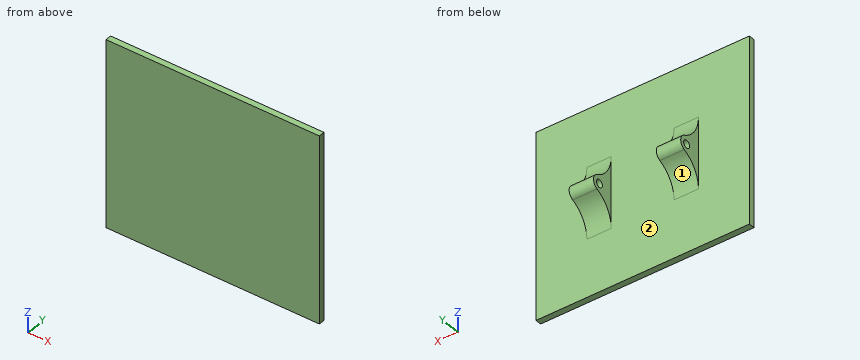
```python
from build123d import *
from build123d.topology import SkipClean

# Parameters (mm, degrees)
SKETCH1_W           = 20
SKETCH1_H           = 60
BOSS_EXTRUDE1_DEPTH = 5
SKETCH2_R           = 2.5
SKETCH2_R_2         = 1.25
BOSS_EXTRUDE2_DEPTH = 20
CUT_EXTRUDE1_START  = -29
SKETCH3_R           = 1.25
CUT_EXTRUDE1_DEPTH  = 29
SKETCH4_R           = 2.5
SKETCH4_R_2         = 1.25
BOSS_EXTRUDE3_DEPTH = 20
CUT_EXTRUDE2_START  = -29
SKETCH5_R           = 1.25
CUT_EXTRUDE2_DEPTH  = 29
BOSS_EXTRUDE4_START = 70
SKETCH7_R           = 1.25
BOSS_EXTRUDE4_DEPTH = 70
SKETCH8_W           = 20.6
SKETCH8_H           = 18.256228475
SKETCH8_W_2         = 16.7
SKETCH8_H_2         = 28.46865204
SKETCH8_H_3         = 26.746757763
CUT_EXTRUDE4_DEPTH  = 84
SKETCH9_W           = 45.88716948
SKETCH9_H           = 69.445914147
CUT_EXTRUDE5_DEPTH  = 115
FILLET1_R           = 10


with BuildPart() as part:
    # Sketch1 → Boss-Extrude1 (new body)
    with BuildSketch(Plane.XY):
        with Locations((10, 30)):
            Rectangle(SKETCH1_W, SKETCH1_H)
    extrude(amount=BOSS_EXTRUDE1_DEPTH)

    # Sketch2 → Boss-Extrude2 (add)
    with BuildSketch(Plane(origin=(20, 0, 0), x_dir=(0, 0, -1), z_dir=(1, 0, 0))):
        with Locations((-2.5, 60)):
            Circle(SKETCH2_R)
        with Locations((-2.5, 60)):
            Circle(SKETCH2_R_2, mode=Mode.SUBTRACT)
    extrude(amount=-BOSS_EXTRUDE2_DEPTH)

    # Sketch3 → Cut-Extrude1 (cut)
    with SkipClean():  # the faces are left unmerged after this step: merging them gives an invalid solid
        with BuildSketch(Plane.ZY.offset(CUT_EXTRUDE1_START)):
            with Locations(Location((2.5, 60, 0), (0, 0, 180))):
                Circle(SKETCH3_R)
        extrude(amount=CUT_EXTRUDE1_DEPTH, mode=Mode.SUBTRACT)

    # Sketch4 → Boss-Extrude3 (add)
    with BuildSketch(Plane.ZY):
        with Locations((2.5, 0)):
            Circle(SKETCH4_R)
        with Locations((2.5, 0)):
            Circle(SKETCH4_R_2, mode=Mode.SUBTRACT)
    extrude(amount=-BOSS_EXTRUDE3_DEPTH)

    # Sketch5 → Cut-Extrude2 (cut)
    with SkipClean():  # the faces are left unmerged after this step: merging them gives an invalid solid
        with BuildSketch(Plane(origin=(20, 0, 0), x_dir=(0, 0, -1), z_dir=(1, 0, 0)).offset(CUT_EXTRUDE2_START)):
            with Locations(Location((-2.5, 0, 0), (0, 0, 180))):
                Circle(SKETCH5_R)
        extrude(amount=CUT_EXTRUDE2_DEPTH, mode=Mode.SUBTRACT)

    # Sketch7 → Boss-Extrude4 (add)
    # profile 1 of 2: a face of its own
    with SkipClean():  # the faces are left unmerged after this step: merging them gives an invalid solid
        with BuildSketch(Plane.ZY.offset(BOSS_EXTRUDE4_START)):
            with BuildLine():
                Line((0, -5), (-27.5, -5))
                Line((-27.5, -5), (-27.5, -7))
                Line((-27.5, -7), (32.5, -7))
                Line((32.5, -7), (32.5, -5))
                Line((32.5, -5), (5, -5))
                Line((5, -5), (5, 0))
                ThreePointArc((5, 0), (2.5, -2.5), (0, 0))
                Line((0, 0), (0, -5))
            make_face()
        # profile 2 of 2: a face of its own
        with BuildSketch(Plane.ZY.offset(BOSS_EXTRUDE4_START)):
            with BuildLine():
                ThreePointArc((5, 0), (2.5, 2.5), (0, 0))
                ThreePointArc((0, 0), (2.5, -2.5), (5, 0))
            make_face()
            with Locations((2.5, 0)):
                Circle(SKETCH7_R, mode=Mode.SUBTRACT)
        extrude(amount=-BOSS_EXTRUDE4_DEPTH)

    # Sketch8 → Cut-Extrude4 (cut)
    with SkipClean():  # the faces are left unmerged after this step: merging them gives an invalid solid
        with BuildSketch(Plane(origin=(0, -5, 0), x_dir=(1, 0, 0), z_dir=(0, 1, 0))):
            with Locations((-35, -1.601019052)):
                Rectangle(SKETCH8_W, SKETCH8_H)
            with Locations((-8.35, -2.689028032)):
                Rectangle(SKETCH8_W_2, SKETCH8_H_2)
            with Locations((-61.65, -3.54997517)):
                Rectangle(SKETCH8_W_2, SKETCH8_H_3)
        extrude(amount=CUT_EXTRUDE4_DEPTH, mode=Mode.SUBTRACT)


with BuildPart() as cut_extrude4_piece_1:
    # of the separate pieces the step leaves, piece 1, a body of its own (cut_extrude4_pieces)
    add(part.part.solids().sort_by_distance((0, -5, 0))[0])

    # Fillet1
    # the kernel refuses this fillet: 10 mm, written as the material it adds along each edge
    with BuildSketch(Plane(origin=(-47.091098093, -5, 5), x_dir=(0, 0, 1), z_dir=(1, 0, 0))) as fillet1_piece_1_section:
        with BuildLine():
            CenterArc((8.956439237, -10), FILLET1_R, 90, 66.421821522)
            Line((-0.208712153, -6), (-1.125227292, -5.6))
            ThreePointArc((-1.125227292, -5.6), (-1, -5), (-1, 0))
            Line((-1, 0), (0, 1))
            Line((0, 1), (8.956439237, 1))
            Line((8.956439237, 1), (8.956439237, 0))
        make_face()
    fillet1_piece_1 = extrude(amount=30.391098093, mode=Mode.PRIVATE)
    fillet1_piece_1 = split(fillet1_piece_1, bisect_by=Plane(origin=(-45.3, -3.872690531, 7.347841943), z_dir=(-1, 0, 0)), keep=Keep.TOP, mode=Mode.PRIVATE)
    add(fillet1_piece_1)
    with BuildSketch(Plane(origin=(-24.7, -5, 5), x_dir=(0, 0, 1), z_dir=(1, 0, 0)), Plane(origin=(-53.3, -5, 5), x_dir=(0, 0, 1), z_dir=(1, 0, 0))) as fillet1_piece_2:
        with BuildLine():
            CenterArc((8.956439237, -10), FILLET1_R, 90, 66.421821522)
            Line((-0.208712153, -6), (-1.125227292, -5.6))
            ThreePointArc((-1.125227292, -5.6), (-1, -5), (-1, 0))
            Line((-1, 0), (0, 1))
            Line((0, 1), (8.956439237, 1))
            Line((8.956439237, 1), (8.956439237, 0))
        make_face()
    extrude(amount=8)
    with BuildSketch(Plane(origin=(-53.3, -5, 5), x_dir=(0, 0, 1), z_dir=(1, 0, 0))) as fillet1_piece_3_section:
        with BuildLine():
            CenterArc((8.956439237, -10), FILLET1_R, 90, 66.421821522)
            Line((-0.208712153, -6), (-1.125227292, -5.6))
            ThreePointArc((-1.125227292, -5.6), (-1, -5), (-1, 0))
            Line((-1, 0), (0, 1))
            Line((0, 1), (8.956439237, 1))
            Line((8.956439237, 1), (8.956439237, 0))
        make_face()
    fillet1_piece_3 = extrude(amount=30.391098093, mode=Mode.PRIVATE)
    fillet1_piece_3 = split(fillet1_piece_3, bisect_by=Plane(origin=(-24.7, -3.872690531, 7.347841943), z_dir=(1, 0, 0)), keep=Keep.TOP, mode=Mode.PRIVATE)
    add(fillet1_piece_3)
    with BuildSketch(Plane(origin=(-53.3, -5, 0), x_dir=(0, 0, -1), z_dir=(1, 0, 0)), Plane(origin=(-24.7, -5, 0), x_dir=(0, 0, -1), z_dir=(1, 0, 0))) as fillet1_piece_4:
        with BuildLine():
            CenterArc((8.956439237, 10), FILLET1_R, 203.578178478, 66.421821522)
            Line((-0.208712153, 6), (-1.125227292, 5.6))
            ThreePointArc((-1.125227292, 5.6), (-1, 5), (-1, 0))
            Line((-1, 0), (0, -1))
            Line((0, -1), (8.956439237, -1))
            Line((8.956439237, -1), (8.956439237, 0))
        make_face()
    extrude(amount=8)
    with BuildSketch(Plane(origin=(-53.3, -5, 0), x_dir=(0, 0, -1), z_dir=(1, 0, 0))) as fillet1_piece_5_section:
        with BuildLine():
            CenterArc((8.956439237, 10), FILLET1_R, 203.578178478, 66.421821522)
            Line((-0.208712153, 6), (-1.125227292, 5.6))
            ThreePointArc((-1.125227292, 5.6), (-1, 5), (-1, 0))
            Line((-1, 0), (0, -1))
            Line((0, -1), (8.956439237, -1))
            Line((8.956439237, -1), (8.956439237, 0))
        make_face()
    fillet1_piece_5 = extrude(amount=30.391098093, mode=Mode.PRIVATE)
    fillet1_piece_5 = split(fillet1_piece_5, bisect_by=Plane(origin=(-24.7, -3.872690531, -2.347841943), z_dir=(1, 0, 0)), keep=Keep.TOP, mode=Mode.PRIVATE)
    add(fillet1_piece_5)
    with BuildSketch(Plane(origin=(-47.091098093, -5, 0), x_dir=(0, 0, -1), z_dir=(1, 0, 0))) as fillet1_piece_6_section:
        with BuildLine():
            CenterArc((8.956439237, 10), FILLET1_R, 203.578178478, 66.421821522)
            Line((-0.208712153, 6), (-1.125227292, 5.6))
            ThreePointArc((-1.125227292, 5.6), (-1, 5), (-1, 0))
            Line((-1, 0), (0, -1))
            Line((0, -1), (8.956439237, -1))
            Line((8.956439237, -1), (8.956439237, 0))
        make_face()
    fillet1_piece_6 = extrude(amount=30.391098093, mode=Mode.PRIVATE)
    fillet1_piece_6 = split(fillet1_piece_6, bisect_by=Plane(origin=(-45.3, -3.872690531, -2.347841943), z_dir=(-1, 0, 0)), keep=Keep.TOP, mode=Mode.PRIVATE)
    add(fillet1_piece_6)


with BuildPart() as cut_extrude4_piece_2:
    # of the separate pieces the step leaves, piece 2, a body of its own (cut_extrude4_pieces)
    add(part.part.solids().sort_by_distance((20, 0, 0))[0])

    # Sketch9 → Cut-Extrude5 (cut)
    with BuildSketch(Plane(origin=(-16.7, 0, 0), x_dir=(0, 0, -1), z_dir=(1, 0, 0))):
        with Locations((-3.398393378, 29.722957074)):
            Rectangle(SKETCH9_W, SKETCH9_H)
    extrude(amount=CUT_EXTRUDE5_DEPTH, mode=Mode.SUBTRACT)


solid = cut_extrude4_piece_1.part
```
Verification items for the finished model (mm, model axes). Face numbers are marked on the shaded views. Give positions to 0.01 mm unless a question says otherwise; leave off trailing zeros. Order: outer loops, then holes, each group sorted by start corner. A loop starts at its lowest first (then second) coordinate and runs counter-clockwise, first axis right, second up. Notation, with made-up numbers: M -24.75,7.25 L 5.25,7.25 A19 ccw 5.25,12.25 Z; hole C -30,48.5 d10. An arc over 180 degrees is marked long. Return JSON: item names as keys, results as strings. Group by question number.
1) Section check D-D on z = 9.5. Record the cut outline in (x, y).
2) Section check A-A on z = 2.5. Record the cut outline in (x, y).
3) Go/stop test with flat-tipped pins: pin 1 Ø2 at (y, z) = (-3, 5) entering from -X; pin 2 Ø4 at (x, y) = (-49, 0) entering from +Z (3 decimals); pin 3 Ø3 at (y, z) = (0, 2.5) entering from +X; pin 4 Ø1.5 at (y, z) = (0, 2.5) entering from +X. Record where each tip stops, or that it passes through.
4) Mould release check, pull along X, two halves, no side actions. Record for the marked faces 1 and 2: pulls with the +X half, pulls with the -X half, needs draft (parallel to the pull), parting line crosses it, or undercut.
5) Section check B-B on y = 0. Record the cut outline in (x, z), and give its area (3 significant figures).
6) Section check C-C on y = -4. Record the cut outline in (x, z).
7) Scan lines: line 1 (X direction, y = -1.75, z = 4); line 2 (Y direction, x = -58.5, z = -25); line 3 (Y direction, x = -51, z = 2). Record each from-to range of solid material in increasing order.
Answer block:
{
 "1": {"outline": "M -70,-7 L 0,-7 L 0,-5 L -16.7,-5 L -16.7,-3.95 L -24.7,-3.95 L -24.7,-5 L -45.3,-5 L -45.3,-3.95 L -53.3,-3.95 L -53.3,-5 L -70,-5 Z"},
 "2": {"outline": "M -70,-7 L 0,-7 L 0,-5 L -16.7,-5 L -16.7,-1.25 L -24.7,-1.25 L -24.7,-5 L -45.3,-5 L -45.3,-1.25 L -53.3,-1.25 L -53.3,-5 L -70,-5 Z; M -53.3,1.25 L -45.3,1.25 L -45.3,2.5 L -53.3,2.5 Z; M -24.7,1.25 L -16.7,1.25 L -16.7,2.5 L -24.7,2.5 Z"},
 "3": {"pin 1": "stops at x = -53.3", "pin 2": "stops at z = 6.815", "pin 3": "stops at x = -16.7", "pin 4": "passes through"},
 "4": {"face 1": "needs draft", "face 2": "undercut"},
 "5": {"outline": "M -53.3,-0.3 L -45.3,-0.3 L -45.3,1.25 L -53.3,1.25 Z; M -53.3,3.75 L -45.3,3.75 L -45.3,5.3 L -53.3,5.3 Z; M -24.7,-0.3 L -16.7,-0.3 L -16.7,1.25 L -24.7,1.25 Z; M -24.7,3.75 L -16.7,3.75 L -16.7,5.3 L -24.7,5.3 Z", "area": "49.5 mm^2"},
 "6": {"outline": "M -53.3,-4.6 L -45.3,-4.6 L -45.3,9.6 L -53.3,9.6 Z; M -24.7,-4.6 L -16.7,-4.6 L -16.7,9.6 L -24.7,9.6 Z"},
 "7": {"line 1": "x = -53.3 to -45.3, -24.7 to -16.7", "line 2": "y = -7 to -5", "line 3": "y = -7 to -1.15, 1.15 to 2.45"}
}
